from build123d import *

# Parameters (mm, degrees)
FILLET1_R       = 0.1
FILLET2_R       = 0.15
HEX_2_DEPTH     = 1.3
THDSCHPAT_COUNT = 13
THDSCHPAT_PITCH = 0.5


with BuildPart() as part:
    # BodySke → Base-Revolve (revolve)
    with BuildSketch(Plane.XY):
        Polygon((0, 0), (0, 2.75), (3, 2.75), (3, 1.5), (10.7195, 1.5), (11, 1.2195), (11, 0), align=None)
    revolve(axis=Axis((-31.75, 0, 0), (1, 0, 0)))

    # Fillet1
    fillet1_edges = [part.edges().sort_by_distance(p)[0] for p in [
        (3, -1.5, 0),
    ]]
    fillet(fillet1_edges, radius=FILLET1_R)

    # Fillet2
    fillet2_edges = [part.edges().sort_by_distance(p)[0] for p in [
        (0, -2.75, 0),
    ]]
    fillet(fillet2_edges, radius=FILLET2_R)

    # Sketch2 → Hex-PreBroach (revolve, cut)
    with BuildSketch(Plane.XY):
        Polygon((0, 1.28), (1.3, 1.28), (2.039008345, 0), (0, 0), align=None)
    revolve(axis=Axis((0, 0, 0), (1, 0, 0)), mode=Mode.SUBTRACT)

    # Sketch3 → Hex 2 (cut)
    with BuildSketch(Plane(origin=(0, 0, 0), x_dir=(0, 0.5, 0.866025404), z_dir=(-1, 0, 0))):
        Polygon((0.739008345, 1.28), (-0.739008345, 1.28), (-1.478016689, 0), (-0.739008345, -1.28), (0.739008345, -1.28), (1.478016689, 0), align=None)
    extrude(amount=-HEX_2_DEPTH, mode=Mode.SUBTRACT)

    # ThdSchSke → ThreadSchematic (revolve, cut)
    with BuildSketch(Plane.XY):
        Polygon((4.5, -1.2195), (4.303591786, -1.5), (4.303591786, -1.875), (4.696408214, -1.875), (4.696408214, -1.5), align=None)
    threadschematic = revolve(axis=Axis((-3.175, 0, 0), (1, 0, 0)), mode=Mode.SUBTRACT)

    # ThdSchPat: ThreadSchematic ×13
    with Locations(*[(i * THDSCHPAT_PITCH, 0, 0) for i in range(1, THDSCHPAT_COUNT)]):
        add(threadschematic, mode=Mode.SUBTRACT)


solid = part.part
Design review of the part built by this model. Coordinates are the model's own, in mm. A direction names the side the tool comes from. Round coordinates to 2 decimals unless told otherwise and drop trailing zeros. One line per question, with ' | ' between items.
(1) Machinability: for faces 1 (the conical face through (1.921, -0.162, -0.124)), 2 (the cylindrical face through (3.71, -1.5, 0.07)), which of the approach directions +Z, -Z, +X, -X, +Y, -Y give a long, thin tool a straight path to every point of the face, cutting with its end or side? Answer none if there is none.
Result sheet:
face 1: -X | face 2: +X
(2) Wall thickness on line 1 (X direction, y = -1.8, z = 0.15); line 2 (Z direction, x = 0.5, y = 0.3); line 3 (X direction, y = -0.2, z = -0.95): over which ranges is each line inside the solid? List them lowest first. Write a range as [from, to].
Result sheet:
line 1: [0, 3] | line 2: [-2.73, -1.28], [1.28, 2.73] | line 3: [1.48, 11]
(3) Draft analysis for pull direction Z (two halves, no side actions). For faces 3 (the flat face through (0.641, -1.114, 0.631)), 4 (the cylindrical face through (1.595, -0.596, -2.685)), state which applies: released by +Z, released by -Z, zero draft, split by the parting line, or undercut.
Result sheet:
face 3: undercut | face 4: split by the parting line
(4) Insertion check: P1, Ø2, axis at x = 9, y = 0.5, coming from the +Z side; P2, Ø0.5, axis at y = -0.5, z = 1, coming from the -X side; P3, Ø1, axis at x = 8.5, z = -1, coming from the -Y side. Each pin has a flat end and moves straight along its axis. Give the tip position at first contact, or say it passes through.
Result sheet:
P1: z = 1.5 | P2: x = 1.3 | P3: y = -1.4
